Build history of the part. All positions in model axes, mm. Face numbers are marked on the shaded views. A direction names the side the tool comes from. Round coordinates to 2 decimals unless told otherwise and drop trailing zeros. Order: outer loops, then holes, each group sorted by start corner. A loop starts at its lowest first (then second) coordinate and runs counter-clockwise, first axis right, second up. Notation, with made-up numbers: (34.25, 67) - (87.25, 67) arc R26 ccw to (87.25, 106) - close; hole circle Ø1 at (4.5, -12). An arc over 180 degrees is marked (long way). Write each question's results on one line, items separated by ' | '. Start each with the question number.
Autodesk Inventor part; units mm, degrees
ref_plane "YZ Plane" through (0, 0, 0) normal (1, 0, 0) x (0, 1, 0)
ref_plane "XZ Plane" through (0, 0, 0) normal (0, 1, 0) x (-1, 0, 0)
ref_plane "XY Plane" through (0, 0, 0) normal (0, 0, 1) x (1, 0, 0)
sketch "スケッチ1" plane through (0, 0, 0) normal (1, 0, 0) x (0, 1, 0)
  line L0 (0, 0) -> (-15, 0)
  line L1 (-15, 0) -> (-15, 15)
  line L2 (-15, 15) -> (0, 15)
  line L3 (0, 15) -> (0, 0)
  line L4 (-13.8, 1.2) -> (-1.2, 1.2)
  line L5 (-1.2, 1.2) -> (-1.2, 13.8)
  line L6 (-1.2, 13.8) -> (-13.8, 13.8)
  line L7 (-13.8, 13.8) -> (-13.8, 1.2)
  dimension "d0" = 15
  dimension "d1" = 15
  dimension "d2" = 1.2
  dimension "d3" = 1.2
  dimension "d4" = 1.2
  dimension "d5" = 1.2
extrude "押し出し1" add sketch "スケッチ1" along normal blind 30
sketch "スケッチ2" plane through (0, -15, 15) normal (0, 0, 1) x (1, 0, 0)
  line L0 (0, 0) -> (30, 0)
  line L1 (30, 15) -> (30, 0)
  point P0 (0, 15)
  point P1 (22.5, 7.5)
  dimension "d8" = 7.5
  dimension "d9" = 7.5
sketch "スケッチ3" plane through (0, 0, 15) normal (0, 1, 0) x (1, 0, 0)
  line L0 (0, 15) -> (0, 0)
  line L1 (0, 15) -> (30, 15)
  point P0 (7.5, 7.5)
  dimension "d10" = 7.5
  dimension "d11" = 7.5
hole "穴1" at (22.5, -7.5, 15) direction (0, 0, -1) diameter 3 end through all
hole "穴2" at (7.5, 0, 7.5) direction (0, -1, 0) diameter 3 end through all
sketch "スケッチ4" plane through (0, -15, 15) normal (0, 0, 1) x (1, 0, 0)
  circle A0 centre (22.5, 7.5) radius 1.5
  line L0 (0, 15) -> (0, 0)
  line L1 (0, 15) -> (30, 15)
  point P0 (11.25, 7.5)
  dimension "d26" = 22.5
  dimension "d27" = 11.25
  dimension "d28" = 7.5
hole "穴3" at (11.25, -7.5, 15) direction (0, 0, -1) diameter 11 end through all
sketch "スケッチ5" plane through (0, 0, 15) normal (0, 1, 0) x (1, 0, 0)
  line L0 (30, 15) -> (30, 0)
  circle A0 centre (7.5, 7.5) radius 1.5
  line L1 (0, 15) -> (30, 15)
  point P0 (18.75, 7.5)
  dimension "d36" = 22.5
  dimension "d37" = 11.25
  dimension "d38" = 7.5
hole "穴4" at (18.75, 0, 7.5) direction (0, -1, 0) diameter 11 end through all
equation "\"d3\" = d2"
equation "\"d4\" = d3"
equation "\"d5\" = d4"
properties part number "ロボットベース15x15x30" material "アルミニウム 6061"
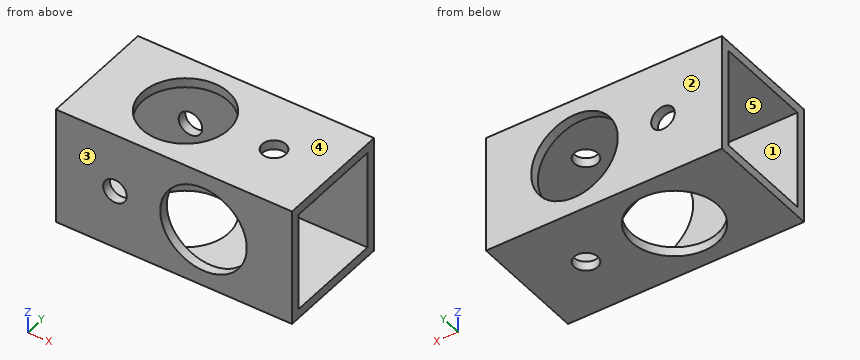
1. Wall check: line 1 (X direction, y = -7.5, z = 0.55); line 2 (Y direction, x = 20.5, z = 2); line 3 (Y direction, x = 22.5, z = 14.15). Give the ranges that are in metal, low to high. Write a range as from..to.
2. Cut at C-C (y = -12). List the corners of the cut face in (x, z), plus the area to 3 significant figures.
3. Mould opens along Z. For the marked faces 3, 4 and 5 say: pulls with the +Z half, pulls with the -Z half, needs draft (parallel to the pull), parting line crosses it, or undercut.
4. 3-axis set-ups, long thin cutter, end or side, ignore diameter. For the marked faces 1 and 2: which of +Z, -Z, +X, -X, +Y, -Y reach the whole face in a straight line?
5. Cut at D-D (z = 13.5). List the corners of the cut face in (x, y), plus the area to 3 significant figures.
6. Cut at B-B (x = 26). List the corners of the cut face in (y, z), plus the area to 3 significant figures.
7. Cut at A-A (z = 7.5). List the corners of the cut face in (x, y).
A:
1) line 1: x = 0..5.75, 16.75..21, 24..30 | line 2: y = -15..-13.8, -1.2..0 | line 3: y = -15..-9, -6..0
2) outline: (0, 0) - (8.09, 0) - (8.09, 1.2) - (0, 1.2) - close; (0, 13.8) - (8.09, 13.8) - (8.09, 15) - (0, 15) - close; (14.41, 0) - (30, 0) - (30, 1.2) - (14.41, 1.2) - close; (14.41, 13.8) - (30, 13.8) - (30, 15) - (14.41, 15) - close | area: 56.8 mm^2
3) face 3: needs draft | face 4: pulls with the +Z half | face 5: undercut
4) face 1: +X, -X | face 2: +Z, -Z, +X, -X, +Y
5) outline: (0, -15) - (30, -15) - (30, -13.8) - (0, -13.8) - close; (0, -1.2) - (30, -1.2) - (30, 0) - (0, 0) - close | area: 72.0 mm^2
6) outline: (-15, 0) - (0, 0) - (0, 15) - (-15, 15) - close; hole (-13.8, 1.2) - (-1.2, 1.2) - (-1.2, 13.8) - (-13.8, 13.8) - close | area: 66.2 mm^2
7) outline: (0, -15) - (6, -15) - (6, -13.8) - (0, -13.8) - close; (0, -1.2) - (6, -1.2) - (6, 0) - (0, 0) - close; (9, -15) - (13.25, -15) - (13.25, -13.8) - (9, -13.8) - close; (9, -1.2) - (13.25, -1.2) - (13.25, 0) - (9, 0) - close; (24.25, -15) - (30, -15) - (30, -13.8) - (24.25, -13.8) - close; (24.25, -1.2) - (30, -1.2) - (30, 0) - (24.25, 0) - close
